The model under review builds one solid part; all positions refer to its coordinate system, in mm. Face numbers are marked on the shaded views. A direction names the side the tool comes from. Coordinates: 2 decimals unless noted, no trailing zeros. Loops run counter-clockwise (first coordinate to the right, second up) from the corner with the lowest first, then second, coordinate; pieces in that order, holes last. Notation, with made-up numbers: M 7,63.5 L 42,63.5 A17 cw 42,79.5 Z; hole C 40.5,11 d11. An arc over 180 degrees is marked long. One line per item, written item: value.
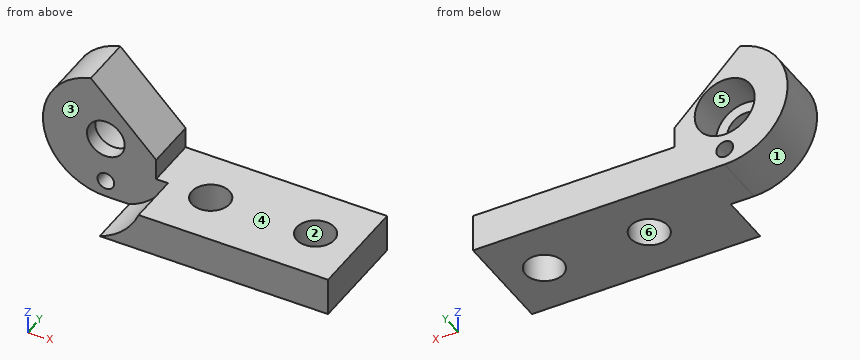
Autodesk Inventor part; units mm, degrees
ref_plane "YZ Plane" through (0, 0, 0) normal (1, 0, 0) x (0, 1, 0)
ref_plane "XZ Plane" through (0, 0, 0) normal (0, 1, 0) x (-1, 0, 0)
ref_plane "XY Plane" through (0, 0, 0) normal (0, 0, 1) x (1, 0, 0)
sketch "Sketch2" plane through (0, 0, 0) normal (0, 1, 0) x (-1, 0, 0)
  line L0 (-60, -6) -> (-60, -15)
  line L1 (-60, -15) -> (0, -15)
  arc A0 (0, -15) -> (3.5692, 14.5692) centre (0, 0) ccw
  line L2 (3.5692, 14.5692) -> (-12, -1)
  line L3 (-12, -1) -> (-12, -6)
  line L4 (-12, -6) -> (-60, -6)
  dimension "d1" = 15
  dimension "d2" = 60
  dimension "d3" = 9
  dimension "d4" = 45
  dimension "d5" = 5
  dimension "d6" = 7.7782
extrude "Extrusion1" add sketch "Sketch2" along normal mid plane 25
sketch "Sketch3" plane through (0, -12.5, 0) normal (0, -1, 0) x (1, 0, 0)
  point P0 (0, 0)
  point P1 (0, 0)
hole "Hole1" at (0, -12.5, 0) direction (0, 1, 0) diameter 32 depth 12.5
sketch "Sketch4" plane through (0, 12.5, 0) normal (0, 1, 0) x (1, 0, 0)
  point P0 (0, 0)
  point P1 (0, 0)
hole "Hole2" at (0, 12.5, 0) direction (0, -1, 0) diameter 9 end through all counterbore diameter 14.3 counterbore depth 9
sketch "Sketch5" plane through (0, 12.5, 0) normal (0, 1, 0) x (1, 0, 0)
  line L0 (0, 0) -> (0, 11) construction
  dimension "d23" = 11
hole "Hole3" at (0, 12.5, -11) direction (0, -1, 0) diameter 4 end through all
sketch "Sketch6" plane through (12, 12.5, -6) normal (0, 0, 1) x (1, 0, 0)
  line L0 (-42, -12.5) -> (63, -12.5) construction
  line L1 (48, -25) -> (48, 0) construction
  point P0 (-12, -12.5)
  point P1 (38, -12.5)
  point P2 (13, -12.5)
  dimension "d31" = 25
  dimension "d32" = 10
hole "Hole4" at (50, 0, -6) at (25, 0, -6) direction (0, 0, -1) diameter 9 end through all
equation "\"d14\" = 0.5 * d7"
equation "\"d21\" = 0.5 * d7"
properties part number "2DU81" material "Aluminum 6061"
(1) Add section C-C on z = -11. State the section outline as (x, y) points.
Checks:
outline: M -10.2,0 L -2,0 L -2,12.5 L -10.2,12.5 Z; M 2,0 L 11.62,0 L 11.62,-12.5 L 60,-12.5 L 60,12.5 L 2,12.5 Z; hole C 25,0 d9; hole C 50,0 d9
(2) Add section D-D on x = 51. State the section outline as (y, z) points.
Checks:
outline: M -12.5,-15 L -4.39,-15 L -4.39,-6 L -12.5,-6 Z; M 4.39,-15 L 12.5,-15 L 12.5,-6 L 4.39,-6 Z
(3) Tool access review of the marked faces 4, 5 and 6: name each direction out of +Z, -Z, +X, -X, +Y, -Y from which nothing blocks a thin tool from reaching the whole face with its end or side.
Checks:
face 4: +Z, +X, +Y, -Y
face 5: +Y
face 6: +Z, -Z
(4) Insertion check: pin 1 Ø8 at (x, y) = (50, 0) entering from +Z; pin 2 Ø14.5 at (x, z) = (0, 0) entering from -Y; pin 3 Ø8 at (x, y) = (-5, 5) entering from +Z; pin 4 Ø10 at (x, z) = (14.5, -2.5) entering from -Y. Each pin has a flat end and moves straight along its axis. Give the tip position at first contact, or say it passes through.
Checks:
pin 1: through
pin 2: y = 0
pin 3: z = 14.57
pin 4: y = -12.5
(5) Draft analysis for pull direction X (two halves, no side actions). For the marked faces 1, 2 and 3, state which applies: pulls with the +X half, pulls with the -X half, needs draft (parallel to the pull), parting line crosses it, or undercut.
Checks:
face 1: pulls with the -X half
face 2: undercut
face 3: needs draft
(6) Add section B-B on z = 0. State the section outline as (x, y) points, then the cut area to 3 significant figures.
Checks:
outline: M -15,0 L -4.5,0 L -4.5,3.5 L -7.15,3.5 L -7.15,12.5 L -15,12.5 Z; M 4.5,0 L 11,0 L 11,12.5 L 7.15,12.5 L 7.15,3.5 L 4.5,3.5 Z
area: 165 mm^2
(7) To check wall thickness, follow L1, parallel to Y at x = 50, z = -9.75; L2, parallel to X at y = -3, z = -12.75; L3, parallel to X at y = -3.25, z = -10. State the ranges of each line that lie inside material, in increasing order. Write a range as [from, to].
Checks:
L1: [-12.5, -4.5], [4.5, 12.5]
L2: [9.67, 21.65], [28.35, 46.65], [53.35, 60]
L3: [12.49, 21.89], [28.11, 46.89], [53.11, 60]
(8) Add section A-A on x = 25. State the section outline as (y, z) points, then the cut area to 3 significant figures.
Checks:
outline: M -12.5,-15 L -4.5,-15 L -4.5,-6 L -12.5,-6 Z; M 4.5,-15 L 12.5,-15 L 12.5,-6 L 4.5,-6 Z
area: 144 mm^2
